from build123d import *

# Parameters (mm, degrees)
SKETCH2_R           = 2
BOSS_EXTRUDE1_DEPTH = 13
SKETCH3_R           = 1.5
BOSS_EXTRUDE2_DEPTH = 7
SKETCH4_W           = 3.988125856
SKETCH4_H           = 4
BOSS_EXTRUDE3_DEPTH = 2
SKETCH5_W           = 2
SKETCH5_H           = 4
BOSS_EXTRUDE4_DEPTH = 7
FILLET1_R           = 2
FILLET2_R           = 2
FILLET3_R           = 2
SKETCH6_R           = 1.5
CUT_EXTRUDE1_DEPTH  = 21.712315177


with BuildPart() as part:
    # Sketch2 → Boss-Extrude1 (new body)
    with BuildSketch(Plane(origin=(0, 0, 0), x_dir=(0, 0, -1), z_dir=(1, 0, 0))):
        Circle(SKETCH2_R)
    extrude(amount=BOSS_EXTRUDE1_DEPTH)

    # Sketch3 → Boss-Extrude2 (add)
    with BuildSketch(Plane(origin=(13, 0, 0), x_dir=(0, 0, -1), z_dir=(1, 0, 0))):
        Circle(SKETCH3_R)
    extrude(amount=BOSS_EXTRUDE2_DEPTH)

    # Sketch4 → Boss-Extrude3 (add)
    with BuildSketch(Plane(origin=(20, 0, 0), x_dir=(0, 0, -1), z_dir=(1, 0, 0))):
        with Locations((-0.005937072, 0)):
            Rectangle(SKETCH4_W, SKETCH4_H)
    extrude(amount=-BOSS_EXTRUDE3_DEPTH)

    # Sketch5 → Boss-Extrude4 (add)
    with BuildSketch(Plane.XY.offset(2)):
        with Locations((19, 0)):
            Rectangle(SKETCH5_W, SKETCH5_H)
    extrude(amount=-BOSS_EXTRUDE4_DEPTH)

    # Fillet1
    fillet1_edges = [part.edges().sort_by_distance(p)[0] for p in [
        (19, 2, 2),
    ]]
    fillet(fillet1_edges, radius=FILLET1_R)

    # Fillet2
    fillet2_edges = [part.edges().sort_by_distance(p)[0] for p in [
        (19, -2, 2),
    ]]
    fillet(fillet2_edges, radius=FILLET2_R - 0.0001)  # a hair under: the kernel refuses the full size

    # Fillet3
    fillet3_edges = [part.edges().sort_by_distance(p)[0] for p in [
        (19, -2, -5),
        (19, 2, -5),
    ]]
    fillet(fillet3_edges, radius=FILLET3_R - 0.0001)  # a hair under: the kernel refuses the full size

    # Sketch6 → Cut-Extrude1 (cut, through all)
    with BuildSketch(Plane(origin=(20, 0, 0), x_dir=(0, 0, -1), z_dir=(1, 0, 0))):
        with Locations((3, 0)):
            Circle(SKETCH6_R)
    extrude(amount=-CUT_EXTRUDE1_DEPTH, mode=Mode.SUBTRACT)


solid = part.part
Here's how the part is built. I have some questions about the finished solid (model axes, mm). A direction names the side the tool comes from. Coordinates: 2 decimals unless noted, no trailing zeros. Write each loop counter-clockwise with the first axis right and the second up, starting at its lowest first coordinate (ties: lowest second). Pieces come first, ordered by that corner, then holes.
1) If I drill on line 1 (X direction, y = -1.05, z = 1.5); line 2 (Y direction, x = 19.55, z = -3); line 3 (Z direction, x = 16.75, y = 0.65), over which ranges is the centre line in solid material (lowest first)?
Filled in:
line 1: x = 0 to 13, 18 to 20
line 2: y = -2 to -1.5, 1.5 to 2
line 3: z = -1.35 to 1.35
2) If we section it at B-B (z = -4): List the corners of the cut face in (x, y) for me, plus the area to 3 significant figures.
Filled in:
outline: (18, -1.73) - (20, -1.73) - (20, -1.12) - (18, -1.12) - close; (18, 1.12) - (20, 1.12) - (20, 1.73) - (18, 1.73) - close
area: 2.46 mm2
3) If we section it at A-A (y = -1.7): List the corners of the cut face in (x, z) for me, plus the area to 3 significant figures.
Filled in:
outline: (0, -1.05) - (13, -1.05) - (13, 1.05) - (0, 1.05) - close; (18, -4.05) - (20, -4.05) - (20, 1.05) - (18, 1.05) - close
area: 37.6 mm2
4) Which directions (+Z, -Z, +X, -X, +Y, -Y) give clear straight access to the entire face, cutting with the end or side of a thin tool? Please do faces 4 (the face through (18, -0.9, -1.5)), 5 (the face through (6.6, 0, -1.5)), 6 (the face through (6, 0, 2)).
Filled in:
face 4: none
face 5: -Z, +X, -X
face 6: -X
5) If we section it at C-C (x = 9): List the corners of the cut face in (y, z) for me, plus the area to 3 significant figures.
Filled in:
outline: (-0.89, -1.79) arc R1.5 cw to (0.89, -1.79) arc R2 ccw (long way) to start
area: 12.0 mm2
6) Thinking about a two-plate mould opening in Y: for faces 1 (the face through (19.014, -0.575, -4.386)), 2 (the face through (19.01, -1.43, -4.4)), 3 (the face through (15.46, 0.07, 1.5)), which applies, +Y half, -Y half, draft (parallel to the pull), parting line (faces both ways), or undercut?
Filled in:
face 1: undercut
face 2: -Y half
face 3: parting line
7) I'm going to push a flat-ended pin straight in: pin 1 (1.5 mm diameter, centred on x = 6.5, y = 0, fed in from -Z). Where does the tip first touch, or does it pass through?
Filled in:
pin 1: stops at z = -1.7
